Autodesk Inventor part; units mm, degrees
ref_plane "dp1_XY" through (12.7, 7.9057, 0) normal (0, 0, 1) x (1, 0, 0)
ref_plane "dp1_YZ" through (12.7, 7.9057, 0) normal (1, 0, 0) x (0, 1, 0)
ref_plane "dp1_ZX" through (12.7, 7.9057, 0) normal (0, 1, 0) x (0, 0, 1)
sketch "Sketch_2" plane through (0, 0, 0) normal (0, 0, 1) x (1, 0, 0)
  line L0 (12.7, 0) -> (0, 0)
  line L1 (0, 0) -> (0, 7.098)
  line L2 (0, 7.098) -> (0.8395, 7.9375)
  line L3 (0.8395, 7.9375) -> (6.6816, 7.9375)
  line L4 (6.6816, 7.9375) -> (7.5202, 7.0965)
  arc A0 (7.5202, 7.0965) -> (8.1407, 6.839) centre (8.1407, 7.7152) ccw
  line L5 (8.1407, 6.839) -> (9.4361, 6.839)
  arc A1 (9.4361, 6.839) -> (10.3124, 7.7153) centre (9.4361, 7.7152) ccw
  line L6 (10.3124, 7.7153) -> (10.3124, 7.9057)
  line L7 (10.3124, 7.9057) -> (12.7, 7.9057)
  line L8 (12.7, 7.9057) -> (12.7, 0)
  line L9 (12.7, 0) -> (0, 0)
revolve "Revolution1" add sketch "Sketch_2" angle 360 about axis through (12.7, 0, 0) along (1, 0, 0)
thread "Thread1"
sketch "Sketch_3" plane through (0, 0, 0) normal (0, 0, 1) x (1, 0, 0)
  line L0 (40.4876, 0) -> (12.7, 0)
  line L1 (12.7, 0) -> (12.7, 10.1918)
  line L2 (12.7, 10.1918) -> (13.462, 10.9537)
  line L3 (13.462, 10.9537) -> (34.0741, 10.9537)
  line L4 (34.0741, 10.9537) -> (34.0741, 8.9091)
  line L5 (34.0741, 8.9091) -> (34.8361, 8.9091)
  line L6 (34.8361, 8.9091) -> (35.5981, 9.671)
  line L7 (35.5981, 9.671) -> (39.7256, 9.671)
  line L8 (39.7256, 9.671) -> (40.4876, 8.9091)
  line L9 (40.4876, 8.9091) -> (40.4876, 0)
  line L10 (40.4876, 0) -> (12.7, 0)
revolve "Revolution2" add sketch "Sketch_3" angle 360 about axis through (40.4876, 0, 0) along (1, 0, 0)
sketch "Sketch3" plane through (0, 0, 0) normal (-1, 0, 0) x (0, 0, 1)
  point P0 (0, 0)
hole "Hole1" at (0, 0, 0) direction (1, 0, 0) diameter 6.4389 depth 40.4876 countersink diameter 6.9469 countersink angle 90
sketch "Sketch_10" plane through (0, 0, 0) normal (0, 0, 1) x (1, 0, 0)
  line L0 (34.0741, 0) -> (30.8991, 0)
  line L1 (30.8991, 15.3353) -> (30.8991, 10.2553)
  line L2 (30.8991, 10.2553) -> (34.0741, 10.2553)
  line L3 (34.0741, 10.2553) -> (34.0741, 15.3353)
  line L4 (34.0741, 15.3353) -> (30.8991, 15.3353)
revolve "Revolution3" cut sketch "Sketch_10" angle 360 about axis through (34.0741, 0, 0) along (1, 0, 0)
sketch "Sketch_43" plane through (0, 0, 0) normal (0, 0, 1) x (1, 0, 0)
  line L0 (24.6126, 0) -> (24.6126, 10.9537)
  line L1 (24.6126, 10.9537) -> (30.0673, 10.9537)
  line L2 (30.0673, 10.9537) -> (29.4323, 10.3187)
  line L3 (29.4323, 10.3187) -> (29.2538, 4.6037)
  line L4 (29.2538, 4.6037) -> (27.7876, 3.7572)
  line L5 (27.7876, 3.7572) -> (27.7876, 0)
  line L6 (27.7876, 0) -> (24.6126, 0)
  line L7 (24.6126, 0) -> (24.6126, 10.9537)
revolve "Revolution4" cut sketch "Sketch_43" angle 360 about axis through (24.6126, 0, 0) along (0, -1, 0)
thread "Thread2"
sketch "Sketch_47" plane through (0, 0, 0) normal (0, 0, 1) x (1, 0, 0)
  line L0 (34.8361, 0) -> (34.0741, 0)
  line L1 (34.0741, 9.512) -> (34.0741, 8.655)
  line L2 (34.0741, 8.655) -> (34.8361, 8.655)
  line L3 (34.8361, 8.655) -> (34.8361, 8.9091)
  line L4 (34.8361, 8.9091) -> (34.4551, 8.9091)
  line L5 (34.4551, 8.9091) -> (34.1966, 9.1676)
  arc A0 (34.1966, 9.3472) -> (34.1966, 9.1676) centre (34.2864, 9.2574) ccw
  line L6 (34.1966, 9.3472) -> (35.0205, 10.1711)
  line L7 (35.0205, 10.1711) -> (35.0205, 10.2553)
  line L8 (35.0205, 10.2553) -> (34.8173, 10.2553)
  line L9 (34.8173, 10.2553) -> (34.0741, 9.512)
revolve "Revolution5" add sketch "Sketch_47" angle 360 about axis through (34.8361, 0, 0) along (1, 0, 0)
ref_plane "dp1_XY" through (12.7, 7.9057, 0) normal (0, 0, 1) x (1, 0, 0)
ref_plane "dp1_YZ" through (12.7, 7.9057, 0) normal (1, 0, 0) x (0, 1, 0)
ref_plane "dp1_ZX" through (12.7, 7.9057, 0) normal (0, 1, 0) x (0, 0, 1)
ref_plane "dp2_XY" through (12.7, -7.9057, 0) normal (0, 0, 1) x (1, 0, 0)
ref_plane "dp2_YZ" through (12.7, -7.9057, 0) normal (1, 0, 0) x (0, 1, 0)
ref_plane "dp2_ZX" through (12.7, -7.9057, 0) normal (0, 1, 0) x (0, 0, 1)
ref_plane "hh_XY" through (0, 7.9375, 0) normal (0, 0, 1) x (1, 0, 0)
ref_plane "hh_YZ" through (0, 7.9375, 0) normal (1, 0, 0) x (0, 1, 0)
ref_plane "hh_ZX" through (0, 7.9375, 0) normal (0, 1, 0) x (0, 0, 1)
ref_plane "port_XY" through (24.6126, 10.9537, 0) normal (0, 0, 1) x (1, 0, 0)
ref_plane "port_YZ" through (24.6126, 10.9537, 0) normal (1, 0, 0) x (0, 1, 0)
ref_plane "port_ZX" through (24.6126, 10.9537, 0) normal (0, 1, 0) x (0, 0, 1)
ref_plane "rod_guide_XY" through (0, 0, 0) normal (1, 0, 0) x (0, 0, -1)
ref_plane "rod_guide_YZ" through (0, 0, 0) normal (0, 0, -1) x (0, 1, 0)
ref_plane "rod_guide_ZX" through (0, 0, 0) normal (0, 1, 0) x (1, 0, 0)
ref_plane "s1_XY" through (10.3124, 0, 0) normal (0, 0, 1) x (1, 0, 0)
ref_plane "s1_YZ" through (10.3124, 0, 0) normal (1, 0, 0) x (0, 1, 0)
ref_plane "s1_ZX" through (10.3124, 0, 0) normal (0, 1, 0) x (0, 0, 1)
ref_plane "s2_XY" through (12.7, 0, 0) normal (0, 0, 1) x (1, 0, 0)
ref_plane "s2_YZ" through (12.7, 0, 0) normal (1, 0, 0) x (0, 1, 0)
ref_plane "s2_ZX" through (12.7, 0, 0) normal (0, 1, 0) x (0, 0, 1)
ref_plane "t1_XY" through (12.7, 0, 0) normal (1, 0, 0) x (0, 0, -1)
ref_plane "t1_YZ" through (12.7, 0, 0) normal (0, 0, -1) x (0, 1, 0)
ref_plane "t1_ZX" through (12.7, 0, 0) normal (0, 1, 0) x (1, 0, 0)
ref_plane "t111_XY" through (12.7, 0, 0) normal (1, 0, 0) x (0, 0, -1)
ref_plane "t111_YZ" through (12.7, 0, 0) normal (0, 0, -1) x (0, 1, 0)
ref_plane "t111_ZX" through (12.7, 0, 0) normal (0, 1, 0) x (1, 0, 0)
ref_plane "to_foot_bracket_XY" through (12.7, 0, 0) normal (1, 0, 0) x (0, 0, -1)
ref_plane "to_foot_bracket_YZ" through (12.7, 0, 0) normal (0, 0, -1) x (0, 1, 0)
ref_plane "to_foot_bracket_ZX" through (12.7, 0, 0) normal (0, 1, 0) x (1, 0, 0)
ref_plane "to_nut_XY" through (10.3124, 0, 0) normal (1, 0, 0) x (0, 0, -1)
ref_plane "to_nut_YZ" through (10.3124, 0, 0) normal (0, 0, -1) x (0, 1, 0)
ref_plane "to_nut_ZX" through (10.3124, 0, 0) normal (0, 1, 0) x (1, 0, 0)
ref_plane "to_rod_XY" through (0, 0, 0) normal (1, 0, 0) x (0, 0, -1)
ref_plane "to_rod_YZ" through (0, 0, 0) normal (0, 0, -1) x (0, 1, 0)
ref_plane "to_rod_ZX" through (0, 0, 0) normal (0, 1, 0) x (1, 0, 0)
ref_plane "to_screw_XY" through (24.6126, -6.0452, -2.032) normal (0, 0, -1) x (1, 0, 0)
ref_plane "to_screw_YZ" through (24.6126, -6.0452, -2.032) normal (1, 0, 0) x (0, -1, 0)
ref_plane "to_screw_ZX" through (24.6126, -6.0452, -2.032) normal (0, -1, 0) x (0, 0, -1)
ref_plane "to_trunnion_brackets_XY" through (11.1252, 0, 0) normal (0, 1, 0) x (1, 0, 0)
ref_plane "to_trunnion_brackets_YZ" through (11.1252, 0, 0) normal (1, 0, 0) x (0, 0, -1)
ref_plane "to_trunnion_brackets_ZX" through (11.1252, 0, 0) normal (0, 0, -1) x (0, 1, 0)
ref_plane "to_trunnion_brackets1_XY" through (11.1252, 12.7, 0) normal (0, 1, 0) x (1, 0, 0)
ref_plane "to_trunnion_brackets1_YZ" through (11.1252, 12.7, 0) normal (1, 0, 0) x (0, 0, -1)
ref_plane "to_trunnion_brackets1_ZX" through (11.1252, 12.7, 0) normal (0, 0, -1) x (0, 1, 0)
ref_plane "to_trunnion_brackets2_XY" through (11.1252, -12.7, 0) normal (0, 1, 0) x (1, 0, 0)
ref_plane "to_trunnion_brackets2_YZ" through (11.1252, -12.7, 0) normal (1, 0, 0) x (0, 0, -1)
ref_plane "to_trunnion_brackets2_ZX" through (11.1252, -12.7, 0) normal (0, 0, -1) x (0, 1, 0)
ref_plane "to_tube_XY" through (34.8361, 0, 0) normal (1, 0, 0) x (0, 0, -1)
ref_plane "to_tube_YZ" through (34.8361, 0, 0) normal (0, 0, -1) x (0, 1, 0)
ref_plane "to_tube_ZX" through (34.8361, 0, 0) normal (0, 1, 0) x (1, 0, 0)
properties part number "04RK000-0_rod_guide"
Verification items for the finished model (mm, model axes). A direction names the side the tool comes from. Give positions to 0.01 mm unless a question says otherwise; leave off trailing zeros. Loops run counter-clockwise (first coordinate to the right, second up) from the corner with the lowest first, then second, coordinate; pieces in that order, holes last.
1. Release check for a two-part mould opening along X. For faces 1 (the cylindrical face through (8.797, 6.523, 2.054)), 2 (the flat face through (30.899, -10, -3)), 3 (the flat face through (0, -3.3, -1.5)), 4 (the conical face through (29.126, 7.501, -1.421)) record: +X half, -X half, draft (parallel to the pull), parting line (faces both ways), or undercut.
Derived:
face 1: undercut
face 2: +X half
face 3: -X half
face 4: undercut
2. Go/stop test with flat-tipped pins: P1, Ø1, axis at y = -5.5, z = 8.5, coming from the -X side; P2, Ø3, axis at x = 26, y = -6.5, coming from the +Z side; P3, Ø1.5, axis at x = 24, y = -7, coming from the -Z side; P4, Ø4, axis at y = 0, z = 0, coming from the +X side. Record where each tip stops, or that it passes through.
Derived:
P1: stops at x = 12.7
P2: stops at z = 9.75
P3: stops at z = -9
P4: passes through
3. Material ranges on probe 1 along Z at (x, y) = (28, 0); probe 2 along Z at (x, y) = (11, 1); probe 3 along X at (y, z) = (8, 1.5), recorded low to high.
Derived:
probe 1: z = -10.95 to -3.22, 3.22 to 10.95
probe 2: z = -7.84 to -3.06, 3.06 to 7.84
probe 3: x = 12.7 to 20.11, 29.12 to 40.49
4. Cross-section at B-B on z = 0. Count the separate pieces of the cut face and the enclosed holes in it, and give its area (3 significant figures).
Derived:
separate pieces: 3
enclosed holes: 0
area: 449 mm2
5. Cross-section at C-C on x = 38. Record the cut outline in (y, z), and give its area (3 significant figures).
Derived:
outline: circle Ø19.34 at (0, 0); hole circle Ø6.44 at (0, 0)
area: 261 mm2
6. Tool access check on faces 5 (the conical face through (29.542, 10.429, 0.06)), 6 (the cylindrical face through (34.648, -1.931, -8.697)), 7 (the cylindrical face through (37.69, -2.1, -9.44)). Record the directions out of +Z, -Z, +X, -X, +Y, -Y that give a thin tool (end or side, any length) a straight path to the whole face; none if there is none.
Derived:
face 5: +Y
face 6: none
face 7: +X
7. Cross-section at A-A on x = 4.5. Record the cut outline in (y, z) (1 decimal), and give its area (3 significant figures).
Derived:
outline: circle Ø15.9 at (0, 0); hole circle Ø6.4 at (0, 0)
area: 165 mm2
